Work out the finished part from the listing and answer in its coordinate system (mm). A direction names the side the tool comes from. Give positions to 0.01 mm unless a question says otherwise; leave off trailing zeros. Write each loop counter-clockwise with the first axis right and the second up, starting at its lowest first coordinate (ties: lowest second). Pieces come first, ordered by that corner, then holes. Notation, with made-up numbers: (30.25, 74.5) - (57.25, 74.5) arc R27 ccw to (57.25, 97.5) - close; hole circle Ø1 at (78, 22.25). An arc over 180 degrees is marked (long way). Write each question's results on one line, items separated by ' | '. Start each with the question number.
from build123d import *

# Parameters (mm, degrees)
SKETCH1_R           = 14
SKETCH1_R_2         = 1.5
BOSS_EXTRUDE1_DEPTH = 32
SKETCH1_3_R         = 1.5
CUT_EXTRUDE1_DEPTH  = 5
SKETCH2_R           = 3
BOSS_EXTRUDE2_DEPTH = 5


with BuildPart() as part:
    # Sketch1 → Boss-Extrude1 (new body)
    # profile 1 of 5: a face of its own
    with BuildSketch(Plane.XY):
        Circle(SKETCH1_R)
        with Locations((0, -8)):
            Circle(SKETCH1_R_2, mode=Mode.SUBTRACT)
        with Locations((0, 8)):
            Circle(SKETCH1_R_2, mode=Mode.SUBTRACT)
        with Locations((-9.5, 0)):
            Circle(SKETCH1_R_2, mode=Mode.SUBTRACT)
        with Locations((9.5, 0)):
            Circle(SKETCH1_R_2, mode=Mode.SUBTRACT)
    # profile 2 of 5: a face of its own
    with BuildSketch(Plane.XY):
        with Locations((-9.5, 0)):
            Circle(SKETCH1_R_2)
    # profile 3 of 5: a face of its own
    with BuildSketch(Plane.XY):
        with Locations((0, 8)):
            Circle(SKETCH1_R_2)
    # profile 4 of 5: a face of its own
    with BuildSketch(Plane.XY):
        with Locations((9.5, 0)):
            Circle(SKETCH1_R_2)
    # profile 5 of 5: a face of its own
    with BuildSketch(Plane.XY):
        with Locations((0, -8)):
            Circle(SKETCH1_R_2)
    extrude(amount=BOSS_EXTRUDE1_DEPTH)

    # Sketch1_3 → Cut-Extrude1 (cut)
    with BuildSketch(Plane.XY):
        with Locations((0, 8)):
            Circle(SKETCH1_3_R)
        with Locations((-9.5, 0)):
            Circle(SKETCH1_3_R)
        with Locations((0, -8)):
            Circle(SKETCH1_3_R)
        with Locations((9.5, 0)):
            Circle(SKETCH1_3_R)
    extrude(amount=CUT_EXTRUDE1_DEPTH, mode=Mode.SUBTRACT)

    # Sketch2 → Boss-Extrude2 (add)
    with BuildSketch(Plane.XY.offset(32)):
        Circle(SKETCH2_R)
    extrude(amount=BOSS_EXTRUDE2_DEPTH)


solid = part.part
Q1. Consider L1, parallel to Y at x = 0, z = 3.15; L2, parallel to Z at x = 0.5, y = -11.5; L3, parallel to Y at x = -9.5, z = 2.7. Determine where each line is inside the solid, lowest interval first.
Q2. A cutting plane is placed at D-D, the plane x = -9.5. Write down the section's boundary in (y, z).
Q3. A cutting plane is placed at C-C, the plane z = 31. Write down the section's boundary in (x, y), and give its area (3 significant figures).
Q4. Given pin 1 (4 mm diameter, centred on x = 0, y = 8, fed in from +Z); pin 2 (5 mm diameter, centred on y = 9, z = 19, fed in from +X); pin 3 (4 mm diameter, centred on x = 0, y = -8, fed in from -Z); pin 4 (0.9 mm diameter, centred on x = 0.5, y = 7.5, fed in from -Z), each flat-ended and moving along its own axis, determine where each tip first touches the part or whether it passes through.
Q5. A cutting plane is placed at B-B, the plane x = 0. Write down the section's boundary in (y, z), and give its area (3 significant figures).
Q6. A tool of negligible diameter and unlimited length cuts with its end or side. For faces 4 (the flat face through (0, 0, 37)), 5 (the cylindrical face through (-11, 0, 2)), from which of +Z, -Z, +X, -X, +Y, -Y can it reach the whole face along a straight path? Write none if from no direction.
Q7. The mould has two halves that part along Y. Classify faces 1 (the flat face through (0, 0, 0)), 2 (the cylindrical face through (-3, 0, 34)), 3 (the flat face through (0, 8, 5)): pulls with the +Y half, pulls with the -Y half, needs draft (parallel to the pull), parting line crosses it, or undercut.
Q8. A cutting plane is placed at A-A, the plane y = 0. Write down the section's boundary in (x, z), and give its area (3 significant figures).
Result:
1) L1: y = -14 to -9.5, -6.5 to 6.5, 9.5 to 14 | L2: z = 0 to 32 | L3: y = -10.28 to -1.5, 1.5 to 10.28
2) outline: (-10.28, 0) - (-1.5, 0) - (-1.5, 5) - (1.5, 5) - (1.5, 0) - (10.28, 0) - (10.28, 32) - (-10.28, 32) - close
3) outline: circle Ø28 at (0, 0) | area: 616 mm2
4) pin 1: stops at z = 32 | pin 2: stops at x = 12.4 | pin 3: stops at z = 0 | pin 4: stops at z = 5
5) outline: (-14, 0) - (-9.5, 0) - (-9.5, 5) - (-6.5, 5) - (-6.5, 0) - (6.5, 0) - (6.5, 5) - (9.5, 5) - (9.5, 0) - (14, 0) - (14, 32) - (3, 32) - (3, 37) - (-3, 37) - (-3, 32) - (-14, 32) - close | area: 896 mm2
6) face 4: +Z, +X, -X, +Y, -Y | face 5: -Z
7) face 1: needs draft | face 2: parting line crosses it | face 3: undercut
8) outline: (-14, 0) - (-11, 0) - (-11, 5) - (-8, 5) - (-8, 0) - (8, 0) - (8, 5) - (11, 5) - (11, 0) - (14, 0) - (14, 32) - (3, 32) - (3, 37) - (-3, 37) - (-3, 32) - (-14, 32) - close | area: 896 mm2
